Design review of the part built by this model. Coordinates are the model's own, in mm. A direction names the side the tool comes from. Give positions to 0.01 mm unless a question says otherwise; leave off trailing zeros. Order: outer loops, then holes, each group sorted by start corner. A loop starts at its lowest first (then second) coordinate and runs counter-clockwise, first axis right, second up. Notation, with made-up numbers: M -20.75,65.5 L 23.25,65.5 A24 ccw 23.25,92.5 Z; hole C -1,6 d2. An arc over 180 degrees is marked long. Answer as a JSON object with one key per item and string values.
from build123d import *

# Parameters (mm, degrees)
SKETCH10_R          = 0.8
SKETCH10_R_2        = 8.3185
BOSS_EXTRUDE1_DEPTH = 4.7625
SKETCH11_W          = 9.525
SKETCH11_H          = 15.875
BOSS_EXTRUDE2_DEPTH = 6.35
FILLET1_R           = 1.905
SKETCH12_R          = 2.667
CUT_EXTRUDE1_DEPTH  = 7.35
FILLET2_R           = 4.445
CHAMFER1_SIZE       = 1.27


with BuildPart() as part:
    # Sketch10 → Boss-Extrude1 (new body)
    with BuildSketch(Plane.XY):
        with BuildLine():
            Line((5.969, 19.548), (5.969, 16.531104381))
            ThreePointArc((5.969, 16.531104381), (5.225051224, 14.735053157), (3.429, 13.991104381))
            Line((3.429, 13.991104381), (-3.429, 13.991104381))
            ThreePointArc((-3.429, 13.991104381), (-5.225051224, 14.735053157), (-5.969, 16.531104381))
            Line((-5.969, 16.531104381), (-5.969, 19.548))
            Line((-5.969, 19.548), (-25.4, 19.548))
            Line((-25.4, 19.548), (-25.4, -3.312))
            Line((-25.4, -3.312), (25.4, -3.312))
            Line((25.4, -3.312), (25.4, 19.548))
            Line((25.4, 19.548), (5.969, 19.548))
        make_face()
        with Locations((21.41, 17.74)):
            Circle(SKETCH10_R, mode=Mode.SUBTRACT)
        with Locations((21.41, 0)):
            Circle(SKETCH10_R, mode=Mode.SUBTRACT)
        with Locations((-21.41, 17.74)):
            Circle(SKETCH10_R, mode=Mode.SUBTRACT)
        with Locations((-21.41, 0)):
            Circle(SKETCH10_R, mode=Mode.SUBTRACT)
        with Locations((13, 8.87)):
            Circle(SKETCH10_R_2, mode=Mode.SUBTRACT)
        with Locations((-13, 8.87)):
            Circle(SKETCH10_R_2, mode=Mode.SUBTRACT)
        with BuildLine():
            Line((-4.7625, 1.5875), (4.7625, 1.5875))
            ThreePointArc((4.7625, 1.5875), (6.35, 0), (4.7625, -1.5875))
            Line((4.7625, -1.5875), (-4.7625, -1.5875))
            ThreePointArc((-4.7625, -1.5875), (-6.35, 0), (-4.7625, 1.5875))
        make_face(mode=Mode.SUBTRACT)
    extrude(amount=BOSS_EXTRUDE1_DEPTH)

    # Sketch11 → Boss-Extrude2 (add)
    with BuildSketch(Plane.XZ.offset(-19.548)):
        with Locations((20.6375, -3.175)):
            Rectangle(SKETCH11_W, SKETCH11_H)
        with Locations((-20.6375, -3.175)):
            Rectangle(SKETCH11_W, SKETCH11_H)
    extrude(amount=-BOSS_EXTRUDE2_DEPTH)

    # Fillet1
    fillet1_edges = [part.edges().sort_by_distance(p)[0] for p in [
        (25.4, -3.312, 2.38125),
        (-25.4, -3.312, 2.38125),
        (-5.969, 19.548, 2.38125),
        (5.969, 19.548, 2.38125),
        (15.875, 19.548, 2.38125),
        (-15.875, 19.548, 2.38125),
    ]]
    fillet(fillet1_edges, radius=FILLET1_R)

    # Sketch12 → Cut-Extrude1 (cut, through all)
    with BuildSketch(Plane.XZ.offset(-19.548)):
        with Locations((-20.6375, -5.55625)):
            Circle(SKETCH12_R)
        with Locations((20.6375, -5.55625)):
            Circle(SKETCH12_R)
    extrude(amount=-CUT_EXTRUDE1_DEPTH, mode=Mode.SUBTRACT)

    # Fillet2
    fillet2_edges = [part.edges().sort_by_distance(p)[0] for p in [
        (25.4, 22.723, -11.1125),
        (15.875, 22.723, -11.1125),
        (-15.875, 22.723, -11.1125),
        (-25.4, 22.723, -11.1125),
    ]]
    fillet(fillet2_edges, radius=FILLET2_R)

    # Chamfer1
    chamfer1_edges = [part.edges().sort_by_distance(p)[0] for p in [
        (-23.3045, 19.548, -5.55625),
        (17.9705, 19.548, -5.55625),
    ]]
    chamfer(chamfer1_edges, length=CHAMFER1_SIZE)


solid = part.part
(1) We need section A-A (x = -13). Write out the cut boundary in (y, z).
Checked values:
{"outline": "M -3.31,0 L 0.55,0 L 0.55,4.76 L -3.31,4.76 Z; M 17.19,0 L 19.55,0 L 19.55,4.76 L 17.19,4.76 Z"}
(2) Insertion check: pin 1 (1.8 mm diameter, centred on x = 21.41, y = 17.74, fed in from -Z); pin 2 (5 mm diameter, centred on x = -12, z = 3, fed in from +Y); pin 3 (5 mm diameter, centred on x = -19.5, z = -6.5, fed in from -Y); pin 4 (6 mm diameter, centred on x = 19.5, y = 9.5, fed in from +Z). Each pin has a flat end and moves straight along its axis. Give the tip position at first contact, or say it passes through.
Checked values:
{"pin 1": "stops at z = 0", "pin 2": "stops at y = 19.62", "pin 3": "stops at y = 19.55", "pin 4": "stops at z = 4.76"}
(3) We need section C-C (z = -0.5). Write out the cut boundary in (x, y) (3 decimals).
Checked values:
{"outline": "M -25.4,19.548 L -15.875,19.548 L -15.875,25.898 L -25.4,25.898 Z; M 15.875,19.548 L 25.4,19.548 L 25.4,25.898 L 15.875,25.898 Z"}
(4) We need section B-B (y = 0). Write out the cut boundary in (x, z), plus the area to 3 significant figures.
Checked values:
{"outline": "M -25.4,0 L -22.21,0 L -22.21,4.76 L -25.4,4.76 Z; M -20.61,0 L -6.35,0 L -6.35,4.76 L -20.61,4.76 Z; M 6.35,0 L 20.61,0 L 20.61,4.76 L 6.35,4.76 Z; M 22.21,0 L 25.4,0 L 25.4,4.76 L 22.21,4.76 Z", "area": "166 mm^2"}
(5) Tool access review of faces 1 (the cylindrical face through (-17.143, 22.767, -9.776)), 2 (the cylindrical face through (-5.21, 14.72, 2.35)), 3 (the flat face through (17, 19.548, -3)), 4 (the flat face through (15.875, 23, -1)): name each direction out of +Z, -Z, +X, -X, +Y, -Y from which nothing blocks a thin tool from reaching the whole face with its end or side.
Checked values:
{"face 1": "-Z, +Y, -Y", "face 2": "+Z, -Z, +Y", "face 3": "-Z, +X, -X, -Y", "face 4": "-Z, +Y"}
(6) To check wall thickness, follow L1, parallel to Y at x = -21.41, z = 3.6; L2, parallel to Y at x = 13, z = 2.95; L3, parallel to X at y = -0.25, z = 0.5. State the ranges of each line that lie inside material, in increasing order. Write a range as from..to.
Checked values:
{"L1": "y = -3.31..-0.8, 0.8..16.94, 18.54..25.9", "L2": "y = -3.31..0.55, 17.19..19.55", "L3": "x = -25.4..-22.17, -20.65..-6.33, 6.33..20.65, 22.17..25.4"}
(7) Draft analysis for pull direction Y (two halves, no side actions). For faces 5 (the flat face through (0, 1.588, 2)), 6 (the flat face through (25.4, 15, 2)), 7 (the flat face through (0, -1.588, 2)), 8 (the cylindrical face through (5.24, 14.75, 2.35)), state which applies: +Y half, -Y half, draft (parallel to the pull), parting line (faces both ways), or undercut.
Checked values:
{"face 5": "undercut", "face 6": "draft", "face 7": "undercut", "face 8": "+Y half"}
(8) We need section D-D (y = 4). Write out the cut boundary in (x, z), plus the area to 3 significant figures.
Checked values:
{"outline": "M -25.4,0 L -19.74,0 L -19.74,4.76 L -25.4,4.76 Z; M -6.26,0 L 6.26,0 L 6.26,4.76 L -6.26,4.76 Z; M 19.74,0 L 25.4,0 L 25.4,4.76 L 19.74,4.76 Z", "area": "113 mm^2"}
